The figure shows three views and two pictorial views of one solid part (mm, origin at its lowest corner). Answer the questions. A direction names the side the tool comes from. Give positions to 0.01 mm unless a question says otherwise; leave off trailing zeros. Write each loop counter-clockwise with the first axis right and the second up, starting at its lowest first coordinate (ties: lowest second). Pieces come first, ordered by that corner, then holes. Notation, with made-up numbers: (-18, -4.75) - (-11, -4.75) arc R29 cw to (-11, 25.25) - close; hole circle Ø2 at (2, -30.5). An arc over 180 degrees is marked (long way). One line per question, with ' | ' between items. Start each with the question number.
1. Given P1, Ø1, axis at y = 35, z = 184.5, coming from the +X side; P2, Ø1.6, axis at x = 15, y = 21, coming from the +Z side; P3, Ø3, axis at x = 6.25, y = 15, coming from the +Z side; P4, Ø3, axis at y = 14, z = 23, coming from the -X side, each flat-ended and moving along its own axis, determine where each tip first touches the part or whether it passes through.
2. Find the intervals of material crossed by L1, parallel to Z at x = 2.25, y = 15; L2, parallel to Y at x = 5, z = 165; L3, parallel to X at y = 20, z = 169, in increasing order. Write a range as from..to.
3. For the marked faces 1 and 2, determine the directions among +Z, -Z, +X, -X, +Y, -Y from which every point of the face is accessible in a straight line to the end or side of a thin tool.
4. A cutting plane is placed at B-B (x = 14.5). Determine the outline of the cut face in (y, z), then the cut area to 3 significant figures.
5. A cutting plane is placed at C-C (y = 54.55). Determine the outline of the cut face in (x, z), then the cut area to 3 significant figures.
6. The mould has two halves that part along Z. Classify the marked faces 3 and 4: +Z half, -Z half, draft (parallel to the pull), parting line (faces both ways), or undercut.
7. A cutting plane is placed at D-D (y = 45). Determine the outline of the cut face in (x, z), then the cut area to 3 significant figures.
8. A cutting plane is placed at A-A (z = 165). Determine the outline of the cut face in (x, y).
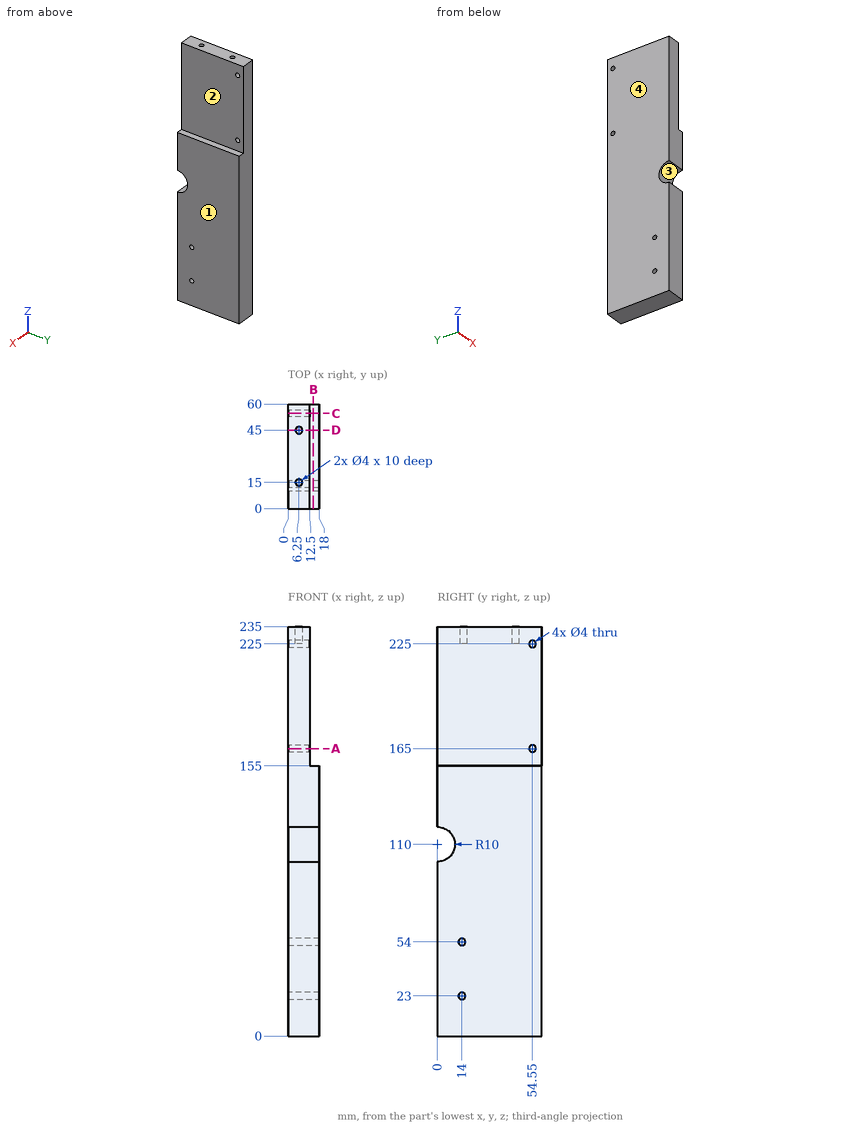
Determined:
1) P1: x = 12.5 | P2: z = 155 | P3: z = 225 | P4: through
2) L1: 0..21.27, 24.73..52.27, 55.73..235 | L2: 0..52.55, 56.55..60 | L3: 0..12.5
3) face 1: +Z, -Z, +X, +Y, -Y | face 2: +Z, +X, +Y, -Y
4) outline: (0, 0) - (60, 0) - (60, 155) - (0, 155) - (0, 120) arc R10 cw to (0, 100) - close; hole circle Ø4 at (14, 23); hole circle Ø4 at (14, 54) | area: 9,120 mm2
5) outline: (0, 0) - (18, 0) - (18, 155) - (12.5, 155) - (12.5, 163) - (0, 163) - close; (0, 167) - (12.5, 167) - (12.5, 223) - (0, 223) - close; (0, 227) - (12.5, 227) - (12.5, 235) - (0, 235) - close | area: 3,690 mm2
6) face 3: undercut | face 4: draft
7) outline: (0, 0) - (18, 0) - (18, 155) - (12.5, 155) - (12.5, 235) - (8.25, 235) - (8.25, 225) - (4.25, 225) - (4.25, 235) - (0, 235) - close | area: 3,750 mm2
8) outline: (0, 0) - (12.5, 0) - (12.5, 52.55) - (0, 52.55) - close; (0, 56.55) - (12.5, 56.55) - (12.5, 60) - (0, 60) - close
